Drawing for the job (mm, zero at the part's lowest x, y, z). A direction names the side the tool comes from. Give positions to 0.01 mm unless a question says otherwise; leave off trailing zeros. Loops run counter-clockwise (first coordinate to the right, second up) from the corner with the lowest first, then second, coordinate; pieces in that order, holes last. Notation, with made-up numbers: (83.25, -23.75) -> (99.25, -23.75) arc R11 cw to (99.25, -9.75) -> close; hole circle Ø10 at (-35, -39.75). An arc over 180 degrees is marked (long way). Use CSV: the item, a comma, the result in double quotes. Start each with the question number.
(1) Cut at A-A on y = 22.5. Write the cut outline in (x, z).
(2) Pull direction X, two halves, no side cores. Call the marked faces 1, 2 and 3: pulls with the +X half, pulls with the -X half, needs draft (parallel to the pull), parting line crosses it, or undercut.
(3) Cut at D-D on x = 15. Write the cut outline in (y, z), then the cut area to 3 significant figures.
(4) Cut at C-C on x = 24.25. Write the cut outline in (y, z).
(5) Drill centre lines: probe 1 along X at (y, z) = (29.5, 4.5); probe 2 along X at (y, z) = (3.5, 5); probe 3 along Z at (x, y) = (24.25, 15). Where is each one in solid material? Low to high.
(6) Flat gauge pins, fed straight in: pin 1 (2.5 mm diameter, centred on x = 5.75, z = 6, fed in from +Y); pin 2 (4 mm diameter, centred on x = 18.5, y = 4.5, fed in from -Z); pin 3 (4.5 mm diameter, centred on x = 15.5, z = 6.5, fed in from -Y). Where does each tip first touch, or does it go through?
(7) 3-axis set-ups, long thin cutter, end or side, ignore diameter. For the marked faces 4 and 5: which of +Z, -Z, +X, -X, +Y, -Y reach the whole face in a straight line?
(8) Cut at B-B on z = 6. Write the cut outline in (x, y), then the cut area to 3 significant figures.
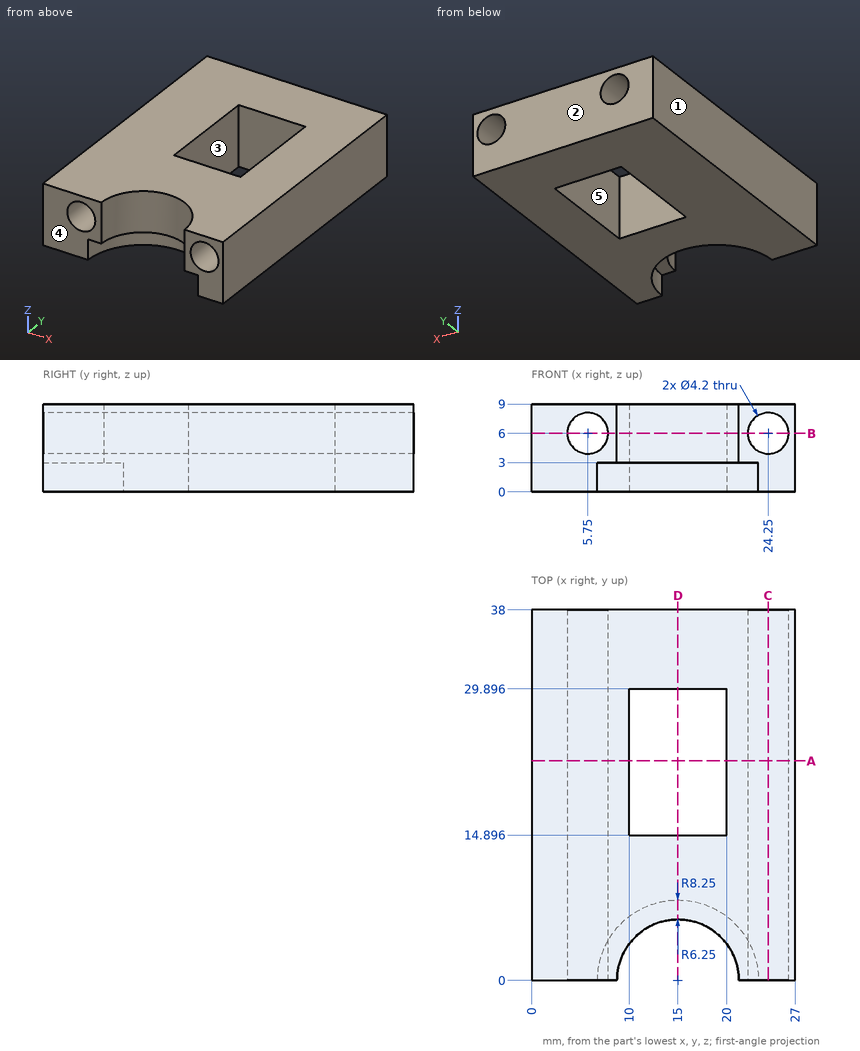
Check result:
1,outline,"(0, 0) -> (10, 0) -> (10, 9) -> (0, 9) -> close; (20, 0) -> (27, 0) -> (27, 9) -> (20, 9) -> close; hole circle Ø4.2 at (5.75, 6); hole circle Ø4.2 at (24.25, 6)"
2,face 1,"pulls with the -X half"
2,face 2,"needs draft"
2,face 3,"undercut"
3,outline,"(6.25, 3) -> (8.25, 3) -> (8.25, 0) -> (14.9, 0) -> (14.9, 9) -> (6.25, 9) -> close; (29.9, 0) -> (38, 0) -> (38, 9) -> (29.9, 9) -> close"
3,area,"145 mm²"
4,outline,"(0, 0) -> (38, 0) -> (38, 3.9) -> (0, 3.9) -> close; (0, 8.1) -> (38, 8.1) -> (38, 9) -> (0, 9) -> close"
5,probe 1,"0 to 4.28, 7.22 to 10, 20 to 22.78, 25.72 to 27"
5,probe 2,"0 to 3.9, 7.6 to 9.82, 20.18 to 22.4, 26.1 to 27"
5,probe 3,"0 to 3.9, 8.1 to 9"
6,pin 1,"through"
6,pin 2,"z = 3"
6,pin 3,"y = 5.61"
7,face 4,"+Z, -Z, +X, -X, -Y"
7,face 5,"+Z, -Z"
8,outline,"(0, 0) -> (3.65, 0) -> (3.65, 38) -> (0, 38) -> close; (7.85, 0) -> (8.75, 0) arc R6.25 cw to (21.25, 0) -> (22.15, 0) -> (22.15, 38) -> (7.85, 38) -> close; (26.35, 0) -> (27, 0) -> (27, 38) -> (26.35, 38) -> close; hole (10, 14.9) -> (20, 14.9) -> (20, 29.9) -> (10, 29.9) -> close"
8,area,"495 mm²"
